from build123d import *

# Parameters (mm, degrees)
SKETCH2_R                = 15.343994309
BOSS_EXTRUDE1_DEPTH      = 21
CUT_EXTRUDE1_DEPTH       = 22
FILLET1_R                = 0.5
CIRPATTERN1_COUNT        = 20
FILLET1_OF_CIRPATTERN1_R = 0.5
CUT_EXTRUDE2_DEPTH       = 22
SKETCH7_R                = 18.5
BOSS_EXTRUDE2_DEPTH      = 1


with BuildPart() as part:
    # Sketch2 → Boss-Extrude1 (new body)
    with BuildSketch(Plane.XY):
        Circle(SKETCH2_R)
    extrude(amount=BOSS_EXTRUDE1_DEPTH)

    # Sketch3 → Cut-Extrude1 (cut, through all)
    with BuildSketch(Plane(origin=(0, 0, 0), x_dir=(-1, 0, 0), z_dir=(0, 0, -1))):
        with BuildLine():
            Line((-1.614471729, 15.258821789), (-1.56, 14.743994309))
            ThreePointArc((-1.56, 14.743994309), (0, 13.183994309), (1.56, 14.743994309))
            Line((1.56, 14.743994309), (1.614471729, 15.258821789))
            ThreePointArc((1.614471729, 15.258821789), (0, 15.343994309), (-1.614471729, 15.258821789))
        make_face()
    cut_extrude1 = extrude(amount=-CUT_EXTRUDE1_DEPTH, mode=Mode.SUBTRACT)

    # Fillet1
    fillet1_edges = [part.edges().sort_by_distance(p)[0] for p in [
        (1.614471729, 15.258821789, 10.5),
        (-1.614471729, 15.258821789, 10.5),
    ]]
    fillet(fillet1_edges, radius=FILLET1_R)

    # CirPattern1: Cut-Extrude1 ×20 about axis
    cirpattern1_axis = Axis((0, 0, 0), (0, 0, 1))
    for i in range(1, CIRPATTERN1_COUNT):
        add(cut_extrude1.rotate(cirpattern1_axis, i * 360 / CIRPATTERN1_COUNT), mode=Mode.SUBTRACT)

    # Fillet1 of CirPattern1
    fillet1_of_cirpattern1_edges = [part.edges().sort_by_distance(p)[0] for p in [
        (-3.179781388, 15.010901095, 10.5),
        (-6.250689106, 14.013102692, 10.5),
        (-7.662775349, 13.293608814, 10.5),
        (-10.275045481, 11.395683469, 10.5),
        (-11.395683469, 10.275045481, 10.5),
        (-13.293608814, 7.662775349, 10.5),
        (-14.013102692, 6.250689106, 10.5),
        (-15.010901095, 3.179781388, 10.5),
        (-15.258821789, 1.614471729, 10.5),
        (-15.258821789, -1.614471729, 10.5),
        (-15.010901095, -3.179781388, 10.5),
        (-14.013102692, -6.250689106, 10.5),
        (-13.293608814, -7.662775349, 10.5),
        (-11.395683469, -10.275045481, 10.5),
        (-10.275045481, -11.395683469, 10.5),
        (-7.662775349, -13.293608814, 10.5),
        (-6.250689106, -14.013102692, 10.5),
        (-3.179781388, -15.010901095, 10.5),
        (-1.614471729, -15.258821789, 10.5),
        (1.614471729, -15.258821789, 10.5),
        (3.179781388, -15.010901095, 10.5),
        (6.250689106, -14.013102692, 10.5),
        (7.662775349, -13.293608814, 10.5),
        (10.275045481, -11.395683469, 10.5),
        (11.395683469, -10.275045481, 10.5),
        (13.293608814, -7.662775349, 10.5),
        (14.013102692, -6.250689106, 10.5),
        (15.010901095, -3.179781388, 10.5),
        (15.258821789, -1.614471729, 10.5),
        (15.258821789, 1.614471729, 10.5),
        (15.010901095, 3.179781388, 10.5),
        (14.013102692, 6.250689106, 10.5),
        (13.293608814, 7.662775349, 10.5),
        (11.395683469, 10.275045481, 10.5),
        (10.275045481, 11.395683469, 10.5),
        (7.662775349, 13.293608814, 10.5),
        (6.250689106, 14.013102692, 10.5),
        (3.179781388, 15.010901095, 10.5),
    ]]
    fillet(fillet1_of_cirpattern1_edges, radius=FILLET1_OF_CIRPATTERN1_R)

    # Sketch5 → Cut-Extrude2 (cut, through all)
    with BuildSketch(Plane(origin=(0, 0, 0), x_dir=(-1, 0, 0), z_dir=(0, 0, -1))):
        with BuildLine():
            Line((-6.3754, 2.527140447), (-6.3754, -2.527140447))
            ThreePointArc((-6.3754, -2.527140447), (-5.939202219, -3.429), (-5.376267826, -4.257688136))
            Line((-5.376267826, -4.257688136), (-0.999132174, -6.784828583))
            ThreePointArc((-0.999132174, -6.784828583), (0, -6.858), (0.999132174, -6.784828583))
            Line((0.999132174, -6.784828583), (5.376267826, -4.257688136))
            ThreePointArc((5.376267826, -4.257688136), (5.939202219, -3.429), (6.3754, -2.527140447))
            Line((6.3754, -2.527140447), (6.3754, 2.527140447))
            ThreePointArc((6.3754, 2.527140447), (5.939202219, 3.429), (5.376267826, 4.257688136))
            Line((5.376267826, 4.257688136), (0.999132174, 6.784828583))
            ThreePointArc((0.999132174, 6.784828583), (0, 6.858), (-0.999132174, 6.784828583))
            Line((-0.999132174, 6.784828583), (-5.376267826, 4.257688136))
            ThreePointArc((-5.376267826, 4.257688136), (-5.939202219, 3.429), (-6.3754, 2.527140447))
        make_face()
    extrude(amount=-CUT_EXTRUDE2_DEPTH, mode=Mode.SUBTRACT)

    # Sketch7 → Boss-Extrude2 (add)
    with BuildSketch(Plane.XY.offset(21)):
        Circle(SKETCH7_R)
        with BuildLine():
            Line((6.3754, -2.527140447), (6.3754, 2.527140447))
            ThreePointArc((6.3754, 2.527140447), (5.939202219, 3.429), (5.376267826, 4.257688136))
            Line((5.376267826, 4.257688136), (0.999132174, 6.784828583))
            ThreePointArc((0.999132174, 6.784828583), (0, 6.858), (-0.999132174, 6.784828583))
            Line((-0.999132174, 6.784828583), (-5.376267826, 4.257688136))
            ThreePointArc((-5.376267826, 4.257688136), (-5.939202219, 3.429), (-6.3754, 2.527140447))
            Line((-6.3754, 2.527140447), (-6.3754, -2.527140447))
            ThreePointArc((-6.3754, -2.527140447), (-5.939202219, -3.429), (-5.376267826, -4.257688136))
            Line((-5.376267826, -4.257688136), (-0.999132174, -6.784828583))
            ThreePointArc((-0.999132174, -6.784828583), (0, -6.858), (0.999132174, -6.784828583))
            Line((0.999132174, -6.784828583), (5.376267826, -4.257688136))
            ThreePointArc((5.376267826, -4.257688136), (5.939202219, -3.429), (6.3754, -2.527140447))
        make_face(mode=Mode.SUBTRACT)
    boss_extrude2 = extrude(amount=BOSS_EXTRUDE2_DEPTH)

    # Mirror1: Boss-Extrude2 across plane
    add(boss_extrude2.mirror(Plane.XY.offset(10.5)))


solid = part.part
Here's how the part is built. I have some questions about the finished solid (model axes, mm). A direction names the side the tool comes from. Coordinates: 2 decimals unless noted, no trailing zeros. Order: outer loops, then holes, each group sorted by start corner. A loop starts at its lowest first (then second) coordinate and runs counter-clockwise, first axis right, second up.
Item 1: If we section it at C-C on x = 9: List the corners of the cut face in (y, z) for me, plus the area to 3 significant figures.
Result sheet:
outline: (-16.16, -1) - (16.16, -1) - (16.16, 0) - (10.4, 0) - (10.4, 21) - (16.16, 21) - (16.16, 22) - (-16.16, 22) - (-16.16, 21) - (-10.4, 21) - (-10.4, 0) - (-16.16, 0) - close
area: 502 mm2
Item 2: For faces 3 (the face through (5.932, -3.441, 10.661)), 4 (the face through (-0.034, -13.184, 10.353)), 5 (the face through (-4.107, -12.528, 10.353)), which set-ups out of +Z, -Z, +X, -X, +Y, -Y let a thin tool reach every point of the face, with its end or its side?
Result sheet:
face 3: +Z, -Z
face 4: -Y
face 5: none
Item 3: If we mould it in two halves opening along Z, with no side actions, what happens to faces 1 (the face through (-3.218, -5.504, 10.661)), 2 (the face through (13.184, -0.034, 10.353))? For each: +Z half, -Z half, draft (parallel to the pull), parting line (faces both ways), or undercut.
Result sheet:
face 1: draft
face 2: undercut
Item 4: If we section it at B-B on y = 0: List the corners of the cut face in (x, z) for me.
Result sheet:
outline: (-18.5, -1) - (-6.38, -1) - (-6.38, 22) - (-18.5, 22) - (-18.5, 21) - (-13.18, 21) - (-13.18, 0) - (-18.5, 0) - close; (6.38, -1) - (18.5, -1) - (18.5, 0) - (13.18, 0) - (13.18, 21) - (18.5, 21) - (18.5, 22) - (6.38, 22) - close
Item 5: For P1, Ø4, axis at x = -9, z = 14, coming from the +Y side; P2, Ø10, axis at x = -3.5, z = 15.5, coming from the +Y side; P3, Ø4, axis at x = -11.5, z = 15, coming from the -Y side, each with a flat end and sliding along its axis, tell me the tip position at first contact or that it passes through.
Result sheet:
P1: stops at y = 13.65
P2: stops at y = 15.2
P3: stops at y = -11.18
Item 6: I need wall thicknesses on line 1 (X direction, y = -1, z = 1.75); line 2 (X direction, y = -13, z = 2.75) (3 decimals); line 3 (Z direction, x = 10.5, y = -14.5). Which ranges of each line are inside material? Lowest first, please.
Result sheet:
line 1: x = -13.55 to -6.38, 6.38 to 13.55
line 2: x = -7.465 to -5.734, -3.378 to 3.378, 5.734 to 7.465
line 3: z = -1 to 0, 21 to 22
Item 7: If we section it at A-A on x = 0: List the corners of the cut face in (y, z) for me, plus the area to 3 significant figures.
Result sheet:
outline: (-18.5, -1) - (-6.86, -1) - (-6.86, 22) - (-18.5, 22) - (-18.5, 21) - (-13.18, 21) - (-13.18, 0) - (-18.5, 0) - close; (6.86, -1) - (18.5, -1) - (18.5, 0) - (13.18, 0) - (13.18, 21) - (18.5, 21) - (18.5, 22) - (6.86, 22) - close
area: 312 mm2
